Design review of the part built by this model. Coordinates are the model's own, in mm. Face numbers are marked on the shaded views. A direction names the side the tool comes from. Give positions to 0.01 mm unless a question says otherwise; leave off trailing zeros. Order: outer loops, then holes, each group sorted by start corner. A loop starts at its lowest first (then second) coordinate and runs counter-clockwise, first axis right, second up. Notation, with made-up numbers: M 62.25,28 L 117.25,28 A12 ccw 117.25,50 Z; hole C 84,80 d7. An arc over 180 degrees is marked long. Put each result on its own line as item: value. Start each with the question number.
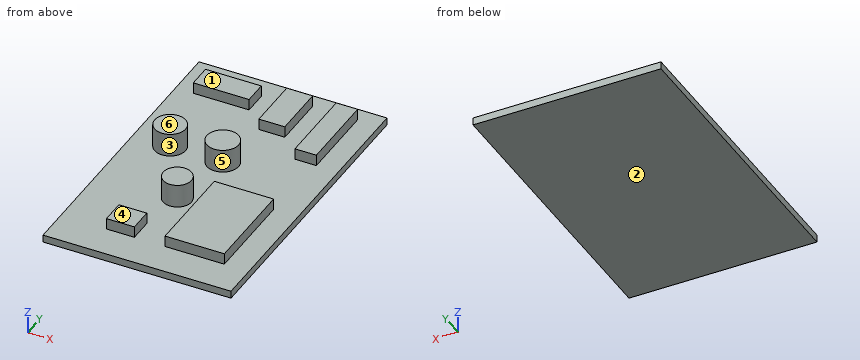
from build123d import *

# Parameters (mm, degrees)
SKETCH1_W           = 25.4
SKETCH1_H           = 40.64
BOSS_EXTRUDE1_DEPTH = 1.016
SKETCH4_R           = 2.089194207
SKETCH4_R_2         = 2.147685622
SKETCH4_R_3         = 1.913924405
BOSS_EXTRUDE3_DEPTH = 3.175
SKETCH3_W           = 2.894795888
SKETCH3_H           = 10.775790564
SKETCH3_W_2         = 3.503459001
SKETCH3_H_2         = 7.272331563
SKETCH3_W_3         = 7.537745123
SKETCH3_H_3         = 3.184962728
SKETCH3_W_4         = 3.768872561
SKETCH3_H_4         = 3.23804544
SKETCH3_W_5         = 8.015489533
SKETCH3_H_5         = 12.846016337
BOSS_EXTRUDE2_DEPTH = 2.54


with BuildPart() as part:
    # Sketch1 → Boss-Extrude1 (new body)
    with BuildSketch(Plane.XY):
        with Locations((-9.742465753, -2.835753425)):
            Rectangle(SKETCH1_W, SKETCH1_H)
    extrude(amount=BOSS_EXTRUDE1_DEPTH)

    # Sketch4 → Boss-Extrude3 (add)
    with BuildSketch(Plane.XY.offset(1.016)):
        with Locations((-17.439459013, 0.322667948)):
            Circle(SKETCH4_R)
        with Locations((-10.326375587, 0.322667948)):
            Circle(SKETCH4_R_2)
        with Locations((-11.706526103, -8.860641252)):
            Circle(SKETCH4_R_3)
    extrude(amount=BOSS_EXTRUDE3_DEPTH)

    # Sketch3 → Boss-Extrude2 (add)
    with BuildSketch(Plane.XY):
        with Locations((-1.447397944, 10.169511049)):
            Rectangle(SKETCH3_W, SKETCH3_H)
        with Locations((-7.831488117, 11.92124055)):
            Rectangle(SKETCH3_W_2, SKETCH3_H_2)
        with Locations((-16.271639347, 12.956353436)):
            Rectangle(SKETCH3_W_3, SKETCH3_H_3)
        with Locations((-14.387203065, -16.902672141)):
            Rectangle(SKETCH3_W_4, SKETCH3_H_4)
        with Locations((-4.354570472, -12.098686692)):
            Rectangle(SKETCH3_W_5, SKETCH3_H_5)
    extrude(amount=BOSS_EXTRUDE2_DEPTH)


solid = part.part
1. Consider section A-A on x = -2.5. Give the boundary of the cut face in (y, z).
2. Insertion check: pin 1 (1.1 mm diameter, centred on x = -8, y = 12, fed in from +Z); pin 2 (0.8 mm diameter, centred on y = 12.5, z = 1.5, fed in from -X); pin 3 (0.5 mm diameter, centred on y = 11, z = 1.5, fed in from -X); pin 4 (1.5 mm diameter, centred on x = -5.5, y = -10.5, fed in from -Z). Each pin has a flat end and moves straight along its axis. Give the tip position at first contact, or say it passes through.
3. Consider section B-B on y = -17. Give the boundary of the cut face in (x, z), then the cut area to 3 significant figures.
4. The part is to be moulded in two halves that separate along X. For the marked faces 5 and 6, say which applies: +X half, -X half, draft (parallel to the pull), parting line (faces both ways), or undercut.
5. Machinability: for the marked faces 1, 2, 3 and 4, which of the approach directions +Z, -Z, +X, -X, +Y, -Y give a long, thin tool a straight path to every point of the face, cutting with its end or side? Answer none if there is none.
6. Consider section D-D on y = 12.5. Give the boundary of the cut face in (x, z).
7. Consider section C-C on z = 1.75. Give the boundary of the cut face in (x, y), then the cut area to 3 significant figures.
8. To check wall thickness, follow probe 1 along Y at (x, z) = (-2.5, 1.6); probe 2 along Z at (x, y) = (1, 3); probe 3 along Z at (x, y) = (-14.75, -18). State the ranges of each line that lie inside material, in increasing order.
Returned:
1. outline: M -23.16,0 L 17.48,0 L 17.48,1.02 L 15.56,1.02 L 15.56,2.54 L 4.78,2.54 L 4.78,1.02 L -5.68,1.02 L -5.68,2.54 L -18.52,2.54 L -18.52,1.02 L -23.16,1.02 Z
2. pin 1: stops at z = 2.54
2. pin 2: stops at x = -20.04
2. pin 3: stops at x = -9.58
2. pin 4: stops at z = 0
3. outline: M -22.44,0 L 2.96,0 L 2.96,1.02 L -0.35,1.02 L -0.35,2.54 L -8.36,2.54 L -8.36,1.02 L -12.5,1.02 L -12.5,2.54 L -16.27,2.54 L -16.27,1.02 L -22.44,1.02 Z
3. area: 43.8 mm2
4. face 5: undercut
4. face 6: draft
5. face 1: +Z, +X, -X, +Y
5. face 2: -Z, +X, -X, +Y, -Y
5. face 3: +Z
5. face 4: +Z, +X, -X, -Y
6. outline: M -22.44,0 L 2.96,0 L 2.96,1.02 L 0,1.02 L 0,2.54 L -2.89,2.54 L -2.89,1.02 L -6.08,1.02 L -6.08,2.54 L -9.58,2.54 L -9.58,1.02 L -12.5,1.02 L -12.5,2.54 L -20.04,2.54 L -20.04,1.02 L -22.44,1.02 Z
7. outline: M -20.04,11.36 L -12.5,11.36 L -12.5,14.55 L -20.04,14.55 Z; C -17.44,0.32 d4.18; M -16.27,-18.52 L -12.5,-18.52 L -12.5,-15.28 L -16.27,-15.28 Z; C -11.71,-8.86 d3.83; C -10.33,0.32 d4.3; M -9.58,8.29 L -6.08,8.29 L -6.08,15.56 L -9.58,15.56 Z; M -8.36,-18.52 L -0.35,-18.52 L -0.35,-5.68 L -8.36,-5.68 Z; M -2.89,4.78 L 0,4.78 L 0,15.56 L -2.89,15.56 Z
7. area: 236 mm2
8. probe 1: y = -18.52 to -5.68, 4.78 to 15.56
8. probe 2: z = 0 to 1.02
8. probe 3: z = 0 to 2.54
